from build123d import *

# Parameters (mm, degrees)
F0_R      = 4.318
F1_DEPTH  = 81.28
F2_R      = 1.778
F3_DEPTH  = 1.27
F5_R      = 7.62
F6_FACE_R = 7.62
F8_R      = 5.08
F10_R     = 8.89
F11_R     = 5.08


with BuildPart() as f1:
    # F0 (on Right) → F1 (new body)
    with BuildSketch(Plane.YZ):
        Circle(F0_R)
    extrude(amount=F1_DEPTH)

    # F2 (on face) → F3 (cut)
    with BuildSketch(Plane.YZ.offset(81.28)):
        Circle(F2_R)
    extrude(amount=-F3_DEPTH, mode=Mode.SUBTRACT)

    # F0 (on Right) → F6 section 0
    with BuildSketch(Plane.YZ):
        Circle(F0_R)
    # F5 (on offset) → F6 section 1
    with BuildSketch(Plane.YZ.offset(-5.08)):
        Circle(F5_R)
    loft()

    # F6_face (on face) → F9 section 0
    with BuildSketch(Plane(origin=(-5.08, 0, 0), x_dir=(0, -1, 0), z_dir=(-1, 0, 0))):
        Circle(F6_FACE_R)
    # F8 (on offset) → F9 section 1
    with BuildSketch(Plane.YZ.offset(-10.16)):
        Circle(F8_R)
    loft()

    # F10
    f10_edges = [f1.edges().sort_by_distance(p)[0] for p in [
        (-5.08, 0, 7.62),
        (-5.08, 0, -7.62),
    ]]
    fillet(f10_edges, radius=F10_R)

    # F11
    f11_edges = [f1.edges().sort_by_distance(p)[0] for p in [
        (0, -4.318, 0),
    ]]
    fillet(f11_edges, radius=F11_R)


solid = f1.part
The model under review builds one solid part; all positions refer to its coordinate system, in mm. Coordinates: 2 decimals unless noted, no trailing zeros. Loops run counter-clockwise (first coordinate to the right, second up) from the corner with the lowest first, then second, coordinate; pieces in that order, holes last. Notation, with made-up numbers: (-13, 11.5) -> (34, 11.5) arc R15 cw to (34, 18.5) -> close; hole circle Ø9 at (-40, -3.75). An arc over 180 degrees is marked (long way). Use a Markdown table: item, result. Add a question column.
1. Draft analysis for pull direction Y (two halves, no side actions). For faces 1 (the face through (-10.16, 0, 0)), 2 (the face through (80.654, -0.385, -1.736)), 3 (the face through (40.824, 4.119, 1.297)), 4 (the face through (80.01, 0, 0)), state which applies: pulls with the +Y half, pulls with the -Y half, needs draft (parallel to the pull), parting line crosses it, or undercut.
2. To check wall thickness, follow line 1 (Z direction, x = 80.6, y = 0); line 2 (Z direction, x = 38.5, y = 0); line 3 (X direction, y = -5, z = -2.5). State the ranges of each line that lie inside material, in increasing order.
3. Clearance check with flat-ended pins moving along their axes: pin 1 Ø5 at (y, z) = (-3, 4.5) entering from +X; pin 2 Ø6 at (x, z) = (43.5, -4.5) entering from +Y; pin 3 Ø3 at (x, z) = (8.5, -2) entering from -Y; pin 4 Ø4 at (x, y) = (20, 2) entering from -Z. State where each tip first meets the part, or that it passes through.
4. Add section A-A on x = 71.5. Write out the cut boundary in (y, z).
Returned:
| question | item | result |
|---|---|---|
| 1 | face 1 | needs draft |
| 1 | face 2 | undercut |
| 1 | face 3 | parting line crosses it |
| 1 | face 4 | undercut |
| 2 | line 1 | z = -4.32 to -1.78, 1.78 to 4.32 |
| 2 | line 2 | z = -4.32 to 4.32 |
| 2 | line 3 | x = -9.1 to -2.22 |
| 3 | pin 1 | stops at x = 81.28 |
| 3 | pin 2 | stops at y = 4.05 |
| 3 | pin 3 | stops at y = -4.29 |
| 3 | pin 4 | stops at z = -4.32 |
| 4 | outline | circle Ø8.64 at (0, 0) |
